Can you work these out from the model? Positions are in its coordinate system, mm. Round coordinates to 2 decimals unless told otherwise and drop trailing zeros. Loops run counter-clockwise (first coordinate to the right, second up) from the corner with the lowest first, then second, coordinate; pieces in that order, holes last.
(1) I want a section at A-A on x = -8. Write out the boundary of the cut face in (y, z) (3 decimals), plus the area to 3 significant figures.
(2) I want a section at C-C on y = 0. Write out the boundary of the cut face in (x, z) (3 decimals), plus the area to 3 significant figures.
(3) Will these pins go through, and if not, where does the flat tip stop? pin 1 Ø1.8 at (x, y) = (-14, 0) entering from +Z; pin 2 Ø1 at (x, z) = (-13, 0.5) entering from -Y.
(4) I want a section at B-B on y = 14. Write out the boundary of the cut face in (x, z).
(5) If I drill on line 1 along Y through (x, z) = (0, 0.7) (3 decimals); line 2 along Y through (x, z) = (-2.5, 1) (3 decimals), over which ranges is the centre line in solid material (lowest first)?
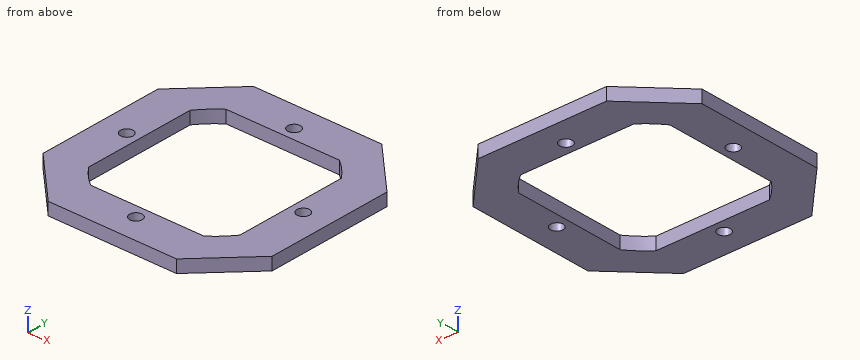
from build123d import *

# Parameters (mm, degrees)
SKETCH_1_R      = 1
EXTRUDE_1_DEPTH = 2


with BuildPart() as part:
    # 草图1 → 凸台-拉伸1 (new body)
    with BuildSketch(Plane.XY):
        Polygon((-18.175, 10.175), (-10.175, 18.175), (10.175, 18.175), (18.175, 10.175), (18.175, -10.175), (10.175, -18.175), (-10.175, -18.175), (-18.175, -10.175), align=None)
        with Locations((0, 14)):
            Circle(SKETCH_1_R, mode=Mode.SUBTRACT)
        with Locations((14, 0)):
            Circle(SKETCH_1_R, mode=Mode.SUBTRACT)
        with Locations((-14, 0)):
            Circle(SKETCH_1_R, mode=Mode.SUBTRACT)
        with Locations((0, -14)):
            Circle(SKETCH_1_R, mode=Mode.SUBTRACT)
        with BuildLine():
            Line((-9, 12), (9, 12))
            ThreePointArc((9, 12), (10.606601718, 10.606601718), (12, 9))
            Line((12, 9), (12, -9))
            ThreePointArc((12, -9), (10.606601718, -10.606601718), (9, -12))
            Line((9, -12), (-9, -12))
            ThreePointArc((-9, -12), (-10.606601718, -10.606601718), (-12, -9))
            Line((-12, -9), (-12, 9))
            ThreePointArc((-12, 9), (-10.606601718, 10.606601718), (-9, 12))
        make_face(mode=Mode.SUBTRACT)
    extrude(amount=EXTRUDE_1_DEPTH)


solid = part.part
Filled sheet:
1. outline: (-18.175, 0) - (-12, 0) - (-12, 2) - (-18.175, 2) - close; (12, 0) - (18.175, 0) - (18.175, 2) - (12, 2) - close
1. area: 24.7 mm2
2. outline: (-18.175, 0) - (-15, 0) - (-15, 2) - (-18.175, 2) - close; (-13, 0) - (-12, 0) - (-12, 2) - (-13, 2) - close; (12, 0) - (13, 0) - (13, 2) - (12, 2) - close; (15, 0) - (18.175, 0) - (18.175, 2) - (15, 2) - close
2. area: 16.7 mm2
3. pin 1: passes through
3. pin 2: stops at y = -15.85
4. outline: (-14.35, 0) - (-1, 0) - (-1, 2) - (-14.35, 2) - close; (1, 0) - (14.35, 0) - (14.35, 2) - (1, 2) - close
5. line 1: y = -18.175 to -15, -13 to -12, 12 to 13, 15 to 18.175
5. line 2: y = -18.175 to -12, 12 to 18.175
